Could you check a few things on this model? Use its own coordinates, in mm. A direction names the side the tool comes from. Coordinates: 2 decimals unless noted, no trailing zeros. Loops run counter-clockwise (first coordinate to the right, second up) from the corner with the lowest first, then second, coordinate; pieces in that order, holes last. Notation, with made-up numbers: M 89,25.5 L 128,25.5 A27 ccw 128,57.5 Z; hole C 66,-12.75 d10. An arc over 180 degrees is marked long. Return JSON: item names as keys, results as strings. Group by question number.
from build123d import *

# Parameters (mm, degrees)
BOSS_EXTRUDE1_DEPTH = 10
SKETCH2_R           = 1.5
CUT_EXTRUDE1_DEPTH  = 10
SKETCH3_R           = 1.5
CUT_EXTRUDE2_DEPTH  = 10
FILLET1_R           = 2


with BuildPart() as part:
    # Sketch1 → Boss-Extrude1 (new body)
    with BuildSketch(Plane.XY):
        Polygon((0, 0), (-14, 0), (-14, -44), (-22.75, -44), (-22.75, -48), (-10, -48), (-10, -4), (0, -4), align=None)
    extrude(amount=BOSS_EXTRUDE1_DEPTH)

    # Sketch2 → Cut-Extrude1 (cut)
    with BuildSketch(Plane(origin=(0, -44, 0), x_dir=(1, 0, 0), z_dir=(0, 1, 0))):
        with Locations(Location((-18.75, -4.25, 0), (0, 0, 270))):
            Circle(SKETCH2_R)
    extrude(amount=-CUT_EXTRUDE1_DEPTH, mode=Mode.SUBTRACT)

    # Sketch3 → Cut-Extrude2 (cut)
    with BuildSketch(Plane(origin=(0, -4, 0), x_dir=(-1, 0, 0), z_dir=(0, -1, 0))):
        with Locations(Location((5, -5, 0), (0, 0, 90))):
            Circle(SKETCH3_R)
    extrude(amount=-CUT_EXTRUDE2_DEPTH, mode=Mode.SUBTRACT)

    # Fillet1
    fillet1_edges = [part.edges().sort_by_distance(p)[0] for p in [
        (0, 0, 5),
    ]]
    fillet(fillet1_edges, radius=FILLET1_R)


solid = part.part
(1) For faces 4 (the face through (-10, -26, 5)), 5 (the face through (-14, -22, 5)), 6 (the face through (0, -3, 5)), which set-ups out of +Z, -Z, +X, -X, +Y, -Y let a thin tool reach every point of the face, with its end or its side?
(2) Imagine slicing it at A-A, the plane x = -5. Write out the boundary of the cut face in (y, z), then the cut area to 3 significant figures.
(3) Imagine slicing it at B-B, the plane z = 9.5. Write out the boundary of the cut face in (x, y), then the cut area to 3 significant figures.
(4) Imagine slicing it at D-D, the plane y = -20. Write out the boundary of the cut face in (x, z), then the cut area to 3 significant figures.
(5) We'd pull the mould along X, two halves only. Please class faces 1 (the face through (-17.485, -45.972, 5.056)), 2 (the face through (-22.75, -46, 5)), 3 (the face through (-8, 0, 5)): +X half, -X half, draft (parallel to the pull), parting line (faces both ways), or undercut.
(6) If I drill on L1, parallel to X at y = -41, z = 4.75; L2, parallel to X at y = -2.95, z = 5; L3, parallel to Y at x = -3.25, z = 4, over which ranges is the centre line in solid material (lowest first)? Write a range as [from, to].
(7) Imagine slicing it at C-C, the plane z = 4.25. Write out the boundary of the cut face in (x, y).
(8) Will these pins go through, and if not, where does the flat tip stop? P1, Ø3, axis at x = -4, z = 7, coming from the -Y side; P2, Ø5, axis at y = -26, z = 5, coming from the -X side; P3, Ø4, axis at y = -28.5, z = 8.5, coming from the +X side.
Checks:
{
 "1": {"face 4": "+Z, -Z, +X, -Y", "face 5": "+Z, -Z, -X, +Y", "face 6": "+Z, -Z, +X, +Y, -Y"},
 "2": {"outline": "M -4,0 L 0,0 L 0,3.5 L -4,3.5 Z; M -4,6.5 L 0,6.5 L 0,10 L -4,10 Z", "area": "28.0 mm²"},
 "3": {"outline": "M -22.75,-48 L -10,-48 L -10,-4 L 0,-4 L 0,-2 A2 ccw -2,0 L -14,0 L -14,-44 L -22.75,-44 Z", "area": "266 mm²"},
 "4": {"outline": "M -14,0 L -10,0 L -10,10 L -14,10 Z", "area": "40.0 mm²"},
 "5": {"face 1": "undercut", "face 2": "-X half", "face 3": "draft"},
 "6": {"L1": "[-14, -10]", "L2": "[-14, -6.5], [-3.5, 0]", "L3": "[-4, 0]"},
 "7": {"outline": "M -22.75,-48 L -20.25,-48 L -20.25,-44 L -22.75,-44 Z; M -17.25,-48 L -10,-48 L -10,-4 L -6.3,-4 L -6.3,0 L -14,0 L -14,-44 L -17.25,-44 Z; M -3.7,-4 L 0,-4 L 0,-2 A2 ccw -2,0 L -3.7,0 Z"},
 "8": {"P1": "y = -4", "P2": "x = -14", "P3": "x = -10"}
}
